```python
from build123d import *

# Parameters (mm, degrees)
ESQUISSE1_W        = 80
ESQUISSE1_H        = 27
BOSS_EXTRU_1_DEPTH = 5
ESQUISSE2_W        = 5
ESQUISSE2_H        = 5
CR_NEAUX_DEPTH     = 5
ESQUISSE3_W        = 10
ESQUISSE3_H        = 5
BOSS_EXTRU_2_DEPTH = 5


with BuildPart() as part:
    # Esquisse1 → Boss.-Extru.1 (new body)
    with BuildSketch(Plane.XY):
        with Locations((161.17461402, 156.921111622)):
            Rectangle(ESQUISSE1_W, ESQUISSE1_H)
    extrude(amount=-BOSS_EXTRU_1_DEPTH)

    # Esquisse2 → Créneaux - (cut)
    with BuildSketch(Plane.XY):
        with Locations((123.67461402, 167.921111622)):
            Rectangle(ESQUISSE2_W, ESQUISSE2_H)
        with Locations((123.67461402, 156.921111622)):
            Rectangle(ESQUISSE2_W, ESQUISSE2_H)
        with Locations((123.67461402, 145.921111622)):
            Rectangle(ESQUISSE2_W, ESQUISSE2_H)
        with Locations((198.67461402, 145.921111622)):
            Rectangle(ESQUISSE2_W, ESQUISSE2_H)
        with Locations((198.67461402, 156.921111622)):
            Rectangle(ESQUISSE2_W, ESQUISSE2_H)
        with Locations((198.67461402, 167.921111622)):
            Rectangle(ESQUISSE2_W, ESQUISSE2_H)
        with BuildLine():
            Line((141.17461402, 162.921111622), (181.17461402, 162.921111622))
            ThreePointArc((181.17461402, 162.921111622), (187.17461402, 156.921111622), (181.17461402, 150.921111622))
            Line((181.17461402, 150.921111622), (141.17461402, 150.921111622))
            ThreePointArc((141.17461402, 150.921111622), (135.17461402, 156.921111622), (141.17461402, 162.921111622))
        make_face()
    extrude(amount=-CR_NEAUX_DEPTH, mode=Mode.SUBTRACT)

    # Esquisse3 → Boss.-Extru.2 (add)
    with BuildSketch(Plane.XY):
        with Locations((138.67461402, 140.921111622)):
            Rectangle(ESQUISSE3_W, ESQUISSE3_H)
        with Locations((171.17461402, 140.921111622)):
            Rectangle(ESQUISSE3_W, ESQUISSE3_H)
    extrude(amount=-BOSS_EXTRU_2_DEPTH)


solid = part.part
```
Verification items for the finished model (mm, model axes). A direction names the side the tool comes from. Coordinates: 2 decimals unless noted, no trailing zeros. Loops run counter-clockwise (first coordinate to the right, second up) from the corner with the lowest first, then second, coordinate; pieces in that order, holes last. Notation, with made-up numbers: (64, 31.5) - (100, 31.5) arc R17 ccw to (100, 51.5) - close; hole circle Ø3 at (72, 71). An arc over 180 degrees is marked (long way). Answer as a JSON object with one key per item and string values.
(1) Cross-section at B-B, the plane x = 160. Record the boundary of the cut face in (y, z).
Response:
{"outline": "(143.42, -5) - (150.92, -5) - (150.92, 0) - (143.42, 0) - close; (162.92, -5) - (170.42, -5) - (170.42, 0) - (162.92, 0) - close"}
(2) Cross-section at A-A, the plane y = 141. Record the boundary of the cut face in (x, z).
Response:
{"outline": "(133.67, -5) - (143.67, -5) - (143.67, 0) - (133.67, 0) - close; (166.17, -5) - (176.17, -5) - (176.17, 0) - (166.17, 0) - close"}
(3) Mould release check, pull along Y, two halves, no side actions. Record for faces 1 (the flat face through (161, 148, -5)), 2 (the flat face through (139, 138.421, -2)), 3 (the flat face through (196.175, 157, -2)): pulls with the +Y half, pulls with the -Y half, needs draft (parallel to the pull), parting line crosses it, or undercut.
Response:
{"face 1": "needs draft", "face 2": "pulls with the -Y half", "face 3": "undercut"}
(4) Cross-section at D-D, the plane x = 188.5. Record the boundary of the cut face in (y, z), then the cut area to 3 significant figures.
Response:
{"outline": "(143.42, -5) - (170.42, -5) - (170.42, 0) - (143.42, 0) - close", "area": "135 mm²"}
(5) Access from +Z, -Z, +X, -X, +Y, -Y to the whole of each face (thin tool, end or side, straight path). Record for faces 4 (the flat face through (199, 165.421, -2)), 5 (the flat face through (166.175, 141, -2)), 6 (the flat face through (124, 154.421, -2)), 7 (the flat face through (126.175, 146, -2)).
Response:
{"face 4": "+Z, -Z, +X, +Y", "face 5": "+Z, -Z, -Y", "face 6": "+Z, -Z, -X", "face 7": "+Z, -Z, -X, -Y"}
(6) Scan lines: line 1 along Y through (x, z) = (145.5, -3.5); line 2 along Y through (x, z) = (170, -1.8); line 3 along Y through (x, z) = (195, -3.6). Record each from-to range of solid material in increasing order.
Response:
{"line 1": "y = 143.42 to 150.92, 162.92 to 170.42", "line 2": "y = 138.42 to 150.92, 162.92 to 170.42", "line 3": "y = 143.42 to 170.42"}
(7) Go/stop test with flat-tipped pins: pin 1 Ø2.5 at (x, z) = (122.5, -3) entering from -Y; pin 2 Ø1.5 at (y, z) = (157, -2) entering from -X; pin 3 Ø1.5 at (y, z) = (140, -2.5) entering from +X. Record where each tip stops, or that it passes through.
Response:
{"pin 1": "stops at y = 148.42", "pin 2": "stops at x = 126.17", "pin 3": "stops at x = 176.17"}
